Verification items for the finished model (mm, model axes). Round coordinates to 2 decimals unless told otherwise and drop trailing zeros. Loops run counter-clockwise (first coordinate to the right, second up) from the corner with the lowest first, then second, coordinate; pieces in that order, holes last. Notation, with made-up numbers: M 68,74.5 L 73,74.5 A35 ccw 73,111.5 Z; hole C 11,44.5 d3. An arc over 180 degrees is marked long. Write item = value, one per line. Start each with the question number.
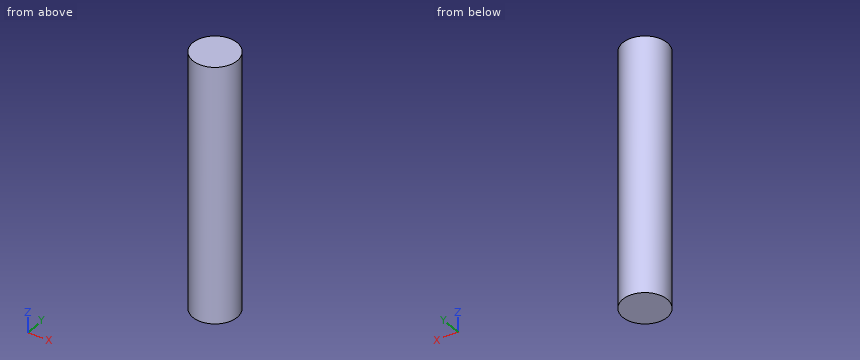
from build123d import *

# Parameters (mm, degrees)
SKETCH1_R               = 2.413
BOSS_EXTRUDE1_DEPTH     = 66.5
SKETCH2_W               = 4.826
SKETCH2_H               = 0.508
CUT_EXTRUDE1_DEPTH      = 6
CUT_EXTRUDE2_DEPTH      = 67.587499863
CUT_EXTRUDE2_DEPTH_BACK = 67.587499863
SKETCH3_W               = 4.826
SKETCH3_H               = 105.06


with BuildPart() as part:
    # Sketch1 → Boss-Extrude1 (new, symmetric)
    with BuildSketch(Plane.XY):
        Circle(SKETCH1_R)
    extrude(amount=BOSS_EXTRUDE1_DEPTH, both=True)

    # Sketch2 → Cut-Extrude1 (cut)
    with BuildSketch(Plane.XY.offset(66.5)):
        with Locations((0, 2.159)):
            Rectangle(SKETCH2_W, SKETCH2_H)
    extrude(amount=-CUT_EXTRUDE1_DEPTH, mode=Mode.SUBTRACT)

    # Sketch3 → Cut-Extrude2 (cut, two sides: drawn at the far end of the back side and taken through both)
    with BuildSketch(Plane(origin=(0, 0, 0), x_dir=(1, 0, 0), z_dir=(0, 1, 0)).offset(-CUT_EXTRUDE2_DEPTH_BACK)):
        with Locations((0, -13.97)):
            Rectangle(SKETCH3_W, SKETCH3_H)
    extrude(amount=CUT_EXTRUDE2_DEPTH + CUT_EXTRUDE2_DEPTH_BACK, mode=Mode.SUBTRACT)


solid = part.part
1. Section check B-B, the plane x = 1.55. Enter the section's corners in (y, z).
2. Thickness scan on line 1 (Y direction, x = 2, z = -65); line 2 (Y direction, x = -0.1, z = -48.5); line 3 (X direction, y = -1.2, z = -45.75). Record the ranges inside material, lowest first.
3. Section check A-A, the plane z = -55.5. Enter the section's corners in (x, y).
4. Section check C-C, the plane y = 1.3. Enter the section's corners in (x, z), and give its area (3 significant figures).
Computed values:
q1.outline = M -1.85,-66.5 L 1.85,-66.5 L 1.85,-38.56 L -1.85,-38.56 Z
q2.line_1 = -1.35 to 1.35
q2.line_2 = -2.41 to 2.41
q2.line_3 = -2.09 to 2.09
q3.outline = C 0,0 d4.83
q4.outline = M -2.03,-66.5 L 2.03,-66.5 L 2.03,-38.56 L -2.03,-38.56 Z
q4.area = 114 mm2
